Geometry: final body of the model. Coordinates: model frame, mm. Coordinates: 2 decimals unless noted, no trailing zeros. Write each loop counter-clockwise with the first axis right and the second up, starting at its lowest first coordinate (ties: lowest second). Pieces come first, ordered by that corner, then holes. Notation, with made-up numbers: (35, 69.5) - (70, 69.5) arc R27 ccw to (70, 97.5) - close; hole circle Ø6 at (-6.5, 31). An arc over 180 degrees is marked (long way). Answer as a JSON object with one key per item and string values. Group by question number.
Item 1: First-contact query: pin 1 Ø5 at (x, z) = (0, 90.5) entering from -Y; pin 2 Ø1 at (y, z) = (4, -25.5) entering from -X; pin 3 Ø6 at (x, z) = (-4, 79) entering from -Y; pin 4 Ø2 at (y, z) = (2, 20.5) entering from +X. Flat tips, straight axial feed; report the tip coordinate or a pass-through.
Item 2: Section C-C on z = 12.5. Return loops of the section in (x, y).
Item 3: Mould query, pull axis X, two halves, no side actions, for faces 1 (the cylindrical face through (0.088, -4.244, 88.502)), 2 (the cylindrical face through (4.77, 1.5, 1.41)). Classes: pulls with the +X half, pulls with the -X half, needs draft (parallel to the pull), parting line crosses it, or undercut.
Item 4: Section B-B on z = 90.5. Return loops of the section in (x, y).
Item 5: Line query: line 1 along Z through (x, y) = (0, 4.5); line 2 along Y through (x, z) = (-0.5, 14.5); line 3 along X through (y, z) = (-0.25, -63). Output: solid intervals per line, ascending. Write a range as from..to.
Item 6: Section A-A on y = 0. Return loops of the section in (x, z).
```python
from build123d import *

# Parameters (mm, degrees)
SKETCH_1_R               = 5
SKETCH_1_R_2             = 4
EXTRUDE_1_DEPTH          = 100.5
CUT_EXTRUDE_1_DEPTH      = 101.74844912
CUT_EXTRUDE_1_DEPTH_BACK = 101.74844912
SKETCH_2_R               = 2


with BuildPart() as part:
    # 草图1 → 凸台-拉伸1 (new, symmetric)
    with BuildSketch(Plane.XY):
        Circle(SKETCH_1_R)
        Circle(SKETCH_1_R_2, mode=Mode.SUBTRACT)
    extrude(amount=EXTRUDE_1_DEPTH, both=True)

    # 草图2 → 切除-拉伸1 (cut, two sides: drawn at the far end of the back side and taken through both)
    with BuildSketch(Plane(origin=(0, 0, 0), x_dir=(1, 0, 0), z_dir=(0, 1, 0)).offset(-CUT_EXTRUDE_1_DEPTH_BACK)):
        with Locations(Location((0, -90.5, 0), (0, 0, 270))):
            Circle(SKETCH_2_R)
        with Locations(Location((0, 90.5, 0), (0, 0, 270))):
            Circle(SKETCH_2_R)
    extrude(amount=CUT_EXTRUDE_1_DEPTH + CUT_EXTRUDE_1_DEPTH_BACK, mode=Mode.SUBTRACT)


solid = part.part
```
Checks:
{
 "1": {"pin 1": "y = -5", "pin 2": "x = -3.57", "pin 3": "y = -4.9", "pin 4": "x = 4.9"},
 "2": {"outline": "circle Ø10 at (0, 0); hole circle Ø8 at (0, 0)"},
 "3": {"face 1": "undercut", "face 2": "parting line crosses it"},
 "4": {"outline": "(-2, -4.58) - (-2, -3.46) arc R4 cw to (-2, 3.46) - (-2, 4.58) arc R5 ccw to start; (2, -4.58) arc R5 ccw to (2, 4.58) - (2, 3.46) arc R4 cw to (2, -3.46) - close"},
 "5": {"line 1": "-100.5..-92.5, -88.5..88.5, 92.5..100.5", "line 2": "-4.97..-3.97, 3.97..4.97", "line 3": "-4.99..-3.99, 3.99..4.99"},
 "6": {"outline": "(-5, -100.5) - (-4, -100.5) - (-4, 100.5) - (-5, 100.5) - close; (4, -100.5) - (5, -100.5) - (5, 100.5) - (4, 100.5) - close"}
}
